For this review, take the finished solid that the model builds, in its own axes (mm). A direction names the side the tool comes from. Round coordinates to 2 decimals unless told otherwise and drop trailing zeros. Loops run counter-clockwise (first coordinate to the right, second up) from the corner with the lowest first, then second, coordinate; pieces in that order, holes last.
1. Tool access review of faces 5 (the flat face through (49, 7, -6)), 6 (the cylindrical face through (45, 6, 51)): name each direction out of +Z, -Z, +X, -X, +Y, -Y from which nothing blocks a thin tool from reaching the whole face with its end or side.
2. Consider section A-A on y = 12.25. State the section outline as (x, z) points.
3. Consider section B-B on x = 53.5. State the section outline as (y, z) points.
4. To check wall thickness, follow line 1 along Z through (x, y) = (27.5, 8); line 2 along Y through (x, z) = (75, 3.5); line 3 along Y through (x, z) = (60, 49). State the ranges of each line that lie inside material, in increasing order.
5. Draft analysis for pull direction X (two halves, no side actions). For faces 1 (the flat face through (49, 0, 48)), 2 (the flat face through (0, 12, 49)), 3 (the flat face through (-6, 7, 46)), 4 (the flat face through (106, 7, 48)), state which applies: released by +X, released by -X, zero draft, split by the parting line, or undercut.
6. Clearance check with flat-ended pins moving along their axes: pin 1 Ø2 at (x, z) = (62, 44) entering from +Y; pin 2 Ø10 at (x, z) = (28.5, 87.5) entering from +Y. State where each tip first meets the part, or that it passes through.
from build123d import *

# Parameters (mm, degrees)
SKETCH1_W           = 100
SKETCH1_H           = 100
BOSS_EXTRUDE1_DEPTH = 10
SKETCH2_W           = 100
SKETCH2_H           = 14
BOSS_EXTRUDE2_DEPTH = 6
SKETCH3_R           = 4
CUT_EXTRUDE1_DEPTH  = 100
FILLET1_DEPTH       = 101
SKETCH4_W           = 106
SKETCH4_H           = 14
BOSS_EXTRUDE3_DEPTH = 6
SKETCH5_W           = 106
SKETCH5_H           = 14
BOSS_EXTRUDE4_DEPTH = 6


with BuildPart() as part:
    # Sketch1 → Boss-Extrude1 (new body)
    with BuildSketch(Plane(origin=(0, 0, 0), x_dir=(1, 0, 0), z_dir=(0, 1, 0))):
        with Locations((50, -50)):
            Rectangle(SKETCH1_W, SKETCH1_H)
    extrude(amount=BOSS_EXTRUDE1_DEPTH)

    # Sketch2 → Boss-Extrude2 (add)
    with BuildSketch(Plane(origin=(0, 0, 0), x_dir=(-1, 0, 0), z_dir=(0, 0, -1))):
        with Locations((-50, 7)):
            Rectangle(SKETCH2_W, SKETCH2_H)
    extrude(amount=BOSS_EXTRUDE2_DEPTH)

    # Sketch3 → Cut-Extrude1 (cut)
    with BuildSketch(Plane.XY.offset(100)):
        with Locations((5, 10)):
            Circle(SKETCH3_R)
        with Locations((15, 10)):
            Circle(SKETCH3_R)
        with Locations((25, 10)):
            Circle(SKETCH3_R)
        with Locations((35, 10)):
            Circle(SKETCH3_R)
        with Locations((45, 10)):
            Circle(SKETCH3_R)
        with Locations((55, 10)):
            Circle(SKETCH3_R)
        with Locations((65, 10)):
            Circle(SKETCH3_R)
        with Locations((75, 10)):
            Circle(SKETCH3_R)
        with Locations((85, 10)):
            Circle(SKETCH3_R)
        with Locations((95, 10)):
            Circle(SKETCH3_R)
    extrude(amount=-CUT_EXTRUDE1_DEPTH, mode=Mode.SUBTRACT)

    # Fillet1: read off the stored shape, not the designer's step
    # Fillet1 outline → Fillet1 (cut)
    with BuildSketch(Plane.XY):
        with BuildLine():
            add(Edge.make_bspline(
                [(1.533333333, 8.004449394), (0.4, 9.973273876), (0, 10)],
                knots=[0, 0, 0, 1, 1, 1], degree=2, weights=[1, 0.881917104, 1]))
            ThreePointArc((1.533333333, 8.004449394), (1.135632868, 8.967204441), (1, 10))
            Line((1, 10), (0, 10))
        make_face()
        with BuildLine():
            add(Edge.make_bspline(
                [(11.535898385, 8), (10.599666447, 9.621601285), (9.99999988, 9.941275628)],
                knots=[0, 0, 0, 0.831887243, 0.831887243, 0.831887243], degree=2, weights=[1, 0.888548242, 0.962527076]))
            ThreePointArc((11.535898385, 8), (11.136296695, 8.96472382), (11, 10))
            Line((11, 10), (9, 10))
            ThreePointArc((9, 10), (8.863703305, 8.96472382), (8.464101615, 8))
            add(Edge.make_bspline(
                [(9.99999988, 9.941275628), (9.400396177, 9.621709752), (8.464101615, 8)],
                knots=[0.168063315, 0.168063315, 0.168063315, 1, 1, 1], degree=2, weights=[0.96253587, 0.888541618, 1]))
        make_face()
        with BuildLine():
            add(Edge.make_bspline(
                [(21.535898385, 8), (20.599666447, 9.621601285), (19.99999988, 9.941275628)],
                knots=[0, 0, 0, 0.831887243, 0.831887243, 0.831887243], degree=2, weights=[1, 0.888548242, 0.962527076]))
            ThreePointArc((21.535898385, 8), (21.136296695, 8.96472382), (21, 10))
            Line((21, 10), (19, 10))
            ThreePointArc((19, 10), (18.863703305, 8.96472382), (18.464101615, 8))
            add(Edge.make_bspline(
                [(19.99999988, 9.941275628), (19.400396177, 9.621709752), (18.464101615, 8)],
                knots=[0.168063315, 0.168063315, 0.168063315, 1, 1, 1], degree=2, weights=[0.96253587, 0.888541618, 1]))
        make_face()
        with BuildLine():
            add(Edge.make_bspline(
                [(31.535898385, 8), (30.599666447, 9.621601285), (29.99999988, 9.941275628)],
                knots=[0, 0, 0, 0.831887243, 0.831887243, 0.831887243], degree=2, weights=[1, 0.888548242, 0.962527076]))
            ThreePointArc((31.535898385, 8), (31.136296695, 8.96472382), (31, 10))
            Line((31, 10), (29, 10))
            ThreePointArc((29, 10), (28.863703305, 8.96472382), (28.464101615, 8))
            add(Edge.make_bspline(
                [(29.99999988, 9.941275628), (29.400396177, 9.621709752), (28.464101615, 8)],
                knots=[0.168063315, 0.168063315, 0.168063315, 1, 1, 1], degree=2, weights=[0.96253587, 0.888541618, 1]))
        make_face()
        with BuildLine():
            add(Edge.make_bspline(
                [(41.535898385, 8), (40.599666447, 9.621601285), (39.99999988, 9.941275628)],
                knots=[0, 0, 0, 0.831887243, 0.831887243, 0.831887243], degree=2, weights=[1, 0.888548242, 0.962527076]))
            ThreePointArc((41.535898385, 8), (41.136296695, 8.96472382), (41, 10))
            Line((41, 10), (39, 10))
            ThreePointArc((39, 10), (38.863703305, 8.96472382), (38.464101615, 8))
            add(Edge.make_bspline(
                [(39.99999988, 9.941275628), (39.400396177, 9.621709752), (38.464101615, 8)],
                knots=[0.168063315, 0.168063315, 0.168063315, 1, 1, 1], degree=2, weights=[0.96253587, 0.888541618, 1]))
        make_face()
        with BuildLine():
            add(Edge.make_bspline(
                [(51.535898385, 8), (50.599666447, 9.621601285), (49.99999988, 9.941275628)],
                knots=[0, 0, 0, 0.831887243, 0.831887243, 0.831887243], degree=2, weights=[1, 0.888548242, 0.962527076]))
            ThreePointArc((51.535898385, 8), (51.136296695, 8.96472382), (51, 10))
            Line((51, 10), (49, 10))
            ThreePointArc((49, 10), (48.863703305, 8.96472382), (48.464101615, 8))
            add(Edge.make_bspline(
                [(49.99999988, 9.941275628), (49.400396177, 9.621709752), (48.464101615, 8)],
                knots=[0.168063315, 0.168063315, 0.168063315, 1, 1, 1], degree=2, weights=[0.96253587, 0.888541618, 1]))
        make_face()
        with BuildLine():
            add(Edge.make_bspline(
                [(61.535898385, 8), (60.599666447, 9.621601285), (59.99999988, 9.941275628)],
                knots=[0, 0, 0, 0.831887243, 0.831887243, 0.831887243], degree=2, weights=[1, 0.888548242, 0.962527076]))
            ThreePointArc((61.535898385, 8), (61.136296695, 8.96472382), (61, 10))
            Line((61, 10), (59, 10))
            ThreePointArc((59, 10), (58.863703305, 8.96472382), (58.464101615, 8))
            add(Edge.make_bspline(
                [(59.99999988, 9.941275628), (59.400396177, 9.621709752), (58.464101615, 8)],
                knots=[0.168063315, 0.168063315, 0.168063315, 1, 1, 1], degree=2, weights=[0.96253587, 0.888541618, 1]))
        make_face()
        with BuildLine():
            add(Edge.make_bspline(
                [(71.535898385, 8), (70.599666447, 9.621601285), (69.99999988, 9.941275628)],
                knots=[0, 0, 0, 0.831887243, 0.831887243, 0.831887243], degree=2, weights=[1, 0.888548242, 0.962527076]))
            ThreePointArc((71.535898385, 8), (71.136296695, 8.96472382), (71, 10))
            Line((71, 10), (69, 10))
            ThreePointArc((69, 10), (68.863703305, 8.96472382), (68.464101615, 8))
            add(Edge.make_bspline(
                [(69.99999988, 9.941275628), (69.400396177, 9.621709752), (68.464101615, 8)],
                knots=[0.168063315, 0.168063315, 0.168063315, 1, 1, 1], degree=2, weights=[0.96253587, 0.888541618, 1]))
        make_face()
        with BuildLine():
            add(Edge.make_bspline(
                [(81.535898385, 8), (80.599666447, 9.621601285), (79.99999988, 9.941275628)],
                knots=[0, 0, 0, 0.831887243, 0.831887243, 0.831887243], degree=2, weights=[1, 0.888548242, 0.962527076]))
            ThreePointArc((81.535898385, 8), (81.136296695, 8.96472382), (81, 10))
            Line((81, 10), (79, 10))
            ThreePointArc((79, 10), (78.863703305, 8.96472382), (78.464101615, 8))
            add(Edge.make_bspline(
                [(79.99999988, 9.941275628), (79.400396177, 9.621709752), (78.464101615, 8)],
                knots=[0.168063315, 0.168063315, 0.168063315, 1, 1, 1], degree=2, weights=[0.96253587, 0.888541618, 1]))
        make_face()
        with BuildLine():
            add(Edge.make_bspline(
                [(91.535898385, 8), (90.599666447, 9.621601285), (89.99999988, 9.941275628)],
                knots=[0, 0, 0, 0.831887243, 0.831887243, 0.831887243], degree=2, weights=[1, 0.888548242, 0.962527076]))
            ThreePointArc((91.535898385, 8), (91.136296695, 8.96472382), (91, 10))
            Line((91, 10), (89, 10))
            ThreePointArc((89, 10), (88.863703305, 8.96472382), (88.464101615, 8))
            add(Edge.make_bspline(
                [(89.99999988, 9.941275628), (89.400396177, 9.621709752), (88.464101615, 8)],
                knots=[0.168063315, 0.168063315, 0.168063315, 1, 1, 1], degree=2, weights=[0.96253587, 0.888541618, 1]))
        make_face()
        with BuildLine():
            add(Edge.make_bspline(
                [(100, 10), (99.6, 9.973273876), (98.466666667, 8.004449394)],
                knots=[0, 0, 0, 1, 1, 1], degree=2, weights=[1, 0.881917104, 1]))
            Line((100, 10), (99, 10))
            ThreePointArc((99, 10), (98.864367132, 8.967204441), (98.466666667, 8.004449394))
        make_face()
    extrude(amount=FILLET1_DEPTH, mode=Mode.SUBTRACT)

    # Sketch4 → Boss-Extrude3 (add)
    with BuildSketch(Plane.ZY):
        with Locations((47, 7)):
            Rectangle(SKETCH4_W, SKETCH4_H)
    extrude(amount=BOSS_EXTRUDE3_DEPTH)

    # Sketch5 → Boss-Extrude4 (add)
    with BuildSketch(Plane(origin=(100, 0, 0), x_dir=(0, 0, -1), z_dir=(1, 0, 0))):
        with Locations((-47, 7)):
            Rectangle(SKETCH5_W, SKETCH5_H)
    extrude(amount=BOSS_EXTRUDE4_DEPTH)


solid = part.part
Resolved:
1. face 5: -Z, +X, -X, +Y, -Y
1. face 6: +Z, +Y
2. outline: (-6, -6) - (106, -6) - (106, 100) - (100, 100) - (100, 0) - (0, 0) - (0, 100) - (-6, 100) - close
3. outline: (0, -6) - (14, -6) - (14, 0) - (6.29, 0) - (6.29, 100) - (0, 100) - close
4. line 1: z = -6 to 0
4. line 2: y = 0 to 6
4. line 3: y = 0 to 9.94
5. face 1: zero draft
5. face 2: undercut
5. face 3: released by -X
5. face 4: released by +X
6. pin 1: stops at y = 8.86
6. pin 2: stops at y = 9.94
